from build123d import *

# Parameters (mm, degrees)
SKETCH2_R                   = 6.35
BOSS_EXTRUDE1_DEPTH         = 6.35
SKETCH3_R                   = 7.9375
BOSS_EXTRUDE2_DEPTH         = 2.54
BOSS_EXTRUDE3_DEPTH         = 1.5875
F_3_8_24_TAPPED_HOLE1_D     = 8.4328
F_3_8_24_TAPPED_HOLE1_DEPTH = 22.352
F_3_8_24_TAPPED_HOLE1_TIP   = 2.533468714
CHAMFER1_SIZE               = 0.254
FILLET1_R                   = 0.79375


with BuildPart() as part:
    # Sketch2 → Boss-Extrude1 (new body)
    with BuildSketch(Plane(origin=(0, 0, 0), x_dir=(1, 0, 0), z_dir=(0, 1, 0))):
        with Locations(Location((0, 0, 0), (0, 0, 270))):
            Circle(SKETCH2_R)
    extrude(amount=BOSS_EXTRUDE1_DEPTH)

    # Sketch3 → Boss-Extrude2 (add)
    with BuildSketch(Plane(origin=(0, 6.35, 0), x_dir=(1, 0, 0), z_dir=(0, 1, 0))):
        with Locations(Location((0, 0, 0), (0, 0, 270))):
            Circle(SKETCH3_R)
    extrude(amount=BOSS_EXTRUDE2_DEPTH)

    # Sketch8 → Boss-Extrude3 (add)
    with BuildSketch(Plane.XZ.offset(-6.35)):
        with BuildLine():
            Line((-0.79375, -6.6675), (-0.79375, 6.6675))
            ThreePointArc((-0.79375, 6.6675), (0, 7.46125), (0.79375, 6.6675))
            Line((0.79375, 6.6675), (0.79375, -6.6675))
            ThreePointArc((0.79375, -6.6675), (0, -7.46125), (-0.79375, -6.6675))
        make_face()
    extrude(amount=BOSS_EXTRUDE3_DEPTH)

    # 3/8-24 Tapped Hole1
    with Locations(Plane(origin=(0, 8.89, 0), x_dir=(-1, 0, 0), z_dir=(0, 1, 0))):
        with Locations((0, 0)):
            Hole(F_3_8_24_TAPPED_HOLE1_D / 2, depth=F_3_8_24_TAPPED_HOLE1_DEPTH)
            with Locations((0, 0, -(F_3_8_24_TAPPED_HOLE1_DEPTH + F_3_8_24_TAPPED_HOLE1_TIP / 2))):  # 118° drill point
                Cone(0, F_3_8_24_TAPPED_HOLE1_D / 2, F_3_8_24_TAPPED_HOLE1_TIP, mode=Mode.SUBTRACT)

    # Chamfer1
    chamfer1_edges = [part.edges().sort_by_distance(p)[0] for p in [
        (0, 0, -6.35),
    ]]
    chamfer(chamfer1_edges, length=CHAMFER1_SIZE)

    # Fillet1
    # the kernel refuses this fillet: 0.79375 mm, written as the material it adds along each edge
    with BuildSketch(Plane(origin=(0.79375, 7.850289674, 6.300195309), x_dir=(0.985141793538893, 0, -0.17174296673509887), z_dir=(0, -1, 0)), Plane(origin=(-0.79375, 7.850289674, -6.300195309), x_dir=(-0.985141793538893, 0, 0.17174296673509887), z_dir=(0, -1, 0))) as fillet1_piece_1:
        with BuildLine():
            CenterArc((0.637623112, 0.792863336), FILLET1_R, 200.939239267, 66.352342207)
            Line((-0.103707592, 0.509194779), (-0.177840663, 0.480827923))
            ThreePointArc((-0.177840663, 0.480827923), (-0.141277627, 0.348215104), (-0.07819563, -0.013632098))
            Line((-0.07819563, -0.013632098), (0.003750724, -0.079286334))
            ThreePointArc((0.003750724, -0.079286334), (0.300057935, -0.072281687), (0.596365145, -0.079286334))
            Line((0.596365145, -0.079286334), (0.60011587, 0))
        make_face()
    extrude(amount=3.087789674)
    with BuildSketch(Plane(origin=(0.79375, 7.850289674, -6.300195309), x_dir=(0.985141793538893, 0, 0.17174296673509887), z_dir=(0, -1, 0)), Plane(origin=(-0.79375, 7.850289674, 6.300195309), x_dir=(-0.985141793538893, 0, -0.17174296673509887), z_dir=(0, -1, 0))) as fillet1_piece_2:
        with BuildLine():
            CenterArc((0.637623112, -0.792863336), FILLET1_R, 92.708418526, 66.352342207)
            Line((-0.103707592, -0.509194779), (-0.177840663, -0.480827923))
            ThreePointArc((-0.177840663, -0.480827923), (-0.141277627, -0.348215104), (-0.07819563, 0.013632098))
            Line((-0.07819563, 0.013632098), (0.003750724, 0.079286334))
            ThreePointArc((0.003750724, 0.079286334), (0.300057935, 0.072281687), (0.596365145, 0.079286334))
            Line((0.596365145, 0.079286334), (0.60011587, 0))
        make_face()
    extrude(amount=3.087789674)


solid = part.part
Design review of the part built by this model. Coordinates are the model's own, in mm. A direction names the side the tool comes from. Give positions to 0.01 mm unless a question says otherwise; leave off trailing zeros. Order: outer loops, then holes, each group sorted by start corner. A loop starts at its lowest first (then second) coordinate and runs counter-clockwise, first axis right, second up. Notation, with made-up numbers: (46, 81) - (64, 81) arc R10 cw to (64, 90) - close; hole circle Ø3 at (-25, 50). An arc over 180 degrees is marked (long way). Write item = value, one per line. Start each with the question number.
Q1. Tool access review of faces 4 (the face through (1.907, 3.259, 6.057)), 5 (the face through (4.15, 0, -1.44)): name each direction out of +Z, -Z, +X, -X, +Y, -Y from which nothing blocks a thin tool from reaching the whole face with its end or side.
Q2. Mouldability with a two-part tool opening along Z and no side actions: class faces 1 (the face through (-3.4, 8.89, 3.4)), 2 (the face through (-7.75, 7.6, -1.72)), 3 (the face through (-0.55, 4.38, 4.18)) as released by +Z, released by -Z, zero draft, split by the parting line, or undercut.
Q3. We need section D-D on y = 7.75. State the section outline as (x, z) points (1 decimal).
Q4. To check wall thickness, follow L1, parallel to Z at x = 0, y = 2; L2, parallel to Y at x = 3, z = 6.25; L3, parallel to X at y = 8, z = 3. State the ranges of each line that lie inside material, in increasing order. Write a range as from..to.
Q5. We need section A-A on y = 5.5. State the section outline as (x, z) points.
Q6. We need section B-B on x = 0. State the section outline as (y, z) points.
Q7. Clearance check with flat-ended pins moving along their axes: pin 1 Ø1 at (x, y) = (-0.5, 1.5) entering from -Z; pin 2 Ø4 at (x, y) = (1.5, 4.5) entering from -Z; pin 3 Ø0.6 at (x, z) = (-0.5, 7) entering from -Y. State where each tip first meets the part, or that it passes through.
Q8. We need section C-C on z = 0. State the section outline as (x, y) points.
Working result:
q1.face_4 = -Y
q1.face_5 = +Z, -Z, +X, -X, -Y
q2.face_1 = zero draft
q2.face_2 = split by the parting line
q2.face_3 = undercut
q3.outline = circle Ø15.9 at (0, 0); hole circle Ø8.4 at (0, 0)
q4.L1 = -6.35..-4.22, 4.22..6.35
q4.L2 = 6.35..8.89
q4.L3 = -7.35..-2.96, 2.96..7.35
q5.outline = (-1.38, -6.2) arc R0.79 cw to (-0.78, -6.82) arc R0.79 ccw to (0.78, -6.82) arc R0.79 cw to (1.38, -6.2) arc R6.35 ccw to (1.38, 6.2) arc R0.79 cw to (0.78, 6.82) arc R0.79 ccw to (-0.78, 6.82) arc R0.79 cw to (-1.38, 6.2) arc R6.35 ccw to start; hole circle Ø8.43 at (0, 0)
q6.outline = (0, -6.1) - (0.25, -6.35) - (4.76, -6.35) - (4.76, -7.46) - (6.35, -7.46) - (6.35, -7.94) - (8.89, -7.94) - (8.89, -4.22) - (0, -4.22) - close; (0, 4.22) - (8.89, 4.22) - (8.89, 7.94) - (6.35, 7.94) - (6.35, 7.46) - (4.76, 7.46) - (4.76, 6.35) - (0.25, 6.35) - (0, 6.1) - close
q7.pin_1 = -6.35
q7.pin_2 = -7.9
q7.pin_3 = 4.76
q8.outline = (-7.94, 6.35) - (-6.35, 6.35) - (-6.35, 0.25) - (-6.1, 0) - (-4.22, 0) - (-4.22, 8.89) - (-7.94, 8.89) - close; (4.22, 0) - (6.1, 0) - (6.35, 0.25) - (6.35, 6.35) - (7.94, 6.35) - (7.94, 8.89) - (4.22, 8.89) - close
